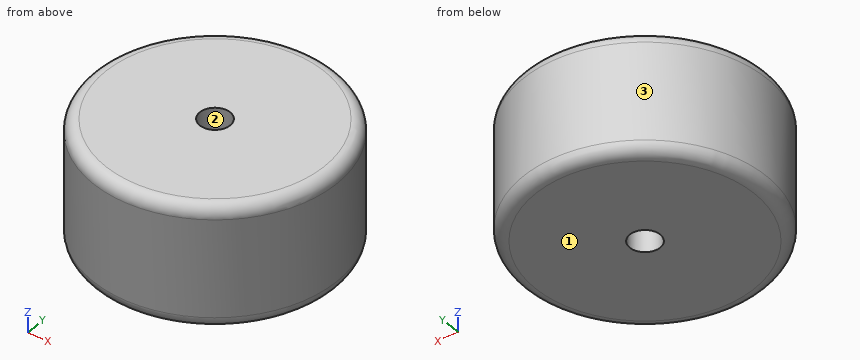
```python
from build123d import *

# Parameters (mm, degrees)
SKETCH1_R           = 25.4
BOSS_EXTRUDE1_DEPTH = 25.4
FILLET1_R           = 2.54
CUT_EXTRUDE1_REACH  = 45.994
SKETCH2_R           = 3.175


with BuildPart() as part:
    # Sketch1 → Boss-Extrude1 (new body)
    with BuildSketch(Plane.XY):
        Circle(SKETCH1_R)
    extrude(amount=BOSS_EXTRUDE1_DEPTH)

    # Fillet1
    fillet1_edges = [part.edges().sort_by_distance(p)[0] for p in [
        (-25.4, 0, 0),
        (-25.4, 0, 25.4),
    ]]
    fillet(fillet1_edges, radius=FILLET1_R)

    # Sketch2 → Cut-Extrude1 (cut, up to next)
    with BuildSketch(Plane.XY.offset(25.4), mode=Mode.PRIVATE) as cut_extrude1_sk1:
        Circle(SKETCH2_R)
    cut_extrude1_tool1 = extrude(cut_extrude1_sk1.sketch, amount=-CUT_EXTRUDE1_REACH, mode=Mode.PRIVATE) & part.part
    add(cut_extrude1_tool1.solids().sort_by_distance((0, 0, 25.4))[0], mode=Mode.SUBTRACT)


solid = part.part
```
Geometry: final body of the model. Coordinates: model frame, mm. Face numbers are marked on the shaded views. Coordinates: 2 decimals unless noted, no trailing zeros. Order: outer loops, then holes, each group sorted by start corner. A loop starts at its lowest first (then second) coordinate and runs counter-clockwise, first axis right, second up. Notation, with made-up numbers: (-23.5, -17.75) - (0.5, -17.75) arc R21 ccw to (0.5, 1.25) - close; hole circle Ø9 at (77, -36). An arc over 180 degrees is marked (long way). Return JSON: item names as keys, results as strings. Group by question number.
1. Cut plane A-A (x = 0). Output: boundary loops of the cut face in (y, z) (3 decimals).
2. Cut plane C-C (z = 10.5). Output: boundary loops of the cut face in (x, y) (3 decimals).
3. Pull-direction query (Y, two-part tool) for the marked faces 1, 2 and 3; classes: pulls with the +Y half, pulls with the -Y half, needs draft (parallel to the pull), parting line crosses it, or undercut.
4. Pin query (flat end, axial travel): pin 1 (4 mm diameter, centred on x = 6, z = 4.5, fed in from -Y); pin 2 (10 mm diameter, centred on y = -15.5, z = 15, fed in from -X); pin 3 (1.5 mm diameter, centred on x = -0.5, z = 14, fed in from +Y). Return the tip coordinate at first contact, or that it passes through.
5. Material intervals for line 1 along Y through (x, z) = (0, 6.75) (3 decimals); line 2 along X through (y, z) = (-2, 21); line 3 along X through (y, z) = (-1.5, 10.75), sorted ascending. Write a range as [from, to].
Resolved:
{
 "1": {"outline": "(-25.4, 2.54) arc R2.54 ccw to (-22.86, 0) - (-3.175, 0) - (-3.175, 25.4) - (-22.86, 25.4) arc R2.54 ccw to (-25.4, 22.86) - close; (3.175, 0) - (22.86, 0) arc R2.54 ccw to (25.4, 2.54) - (25.4, 22.86) arc R2.54 ccw to (22.86, 25.4) - (3.175, 25.4) - close"},
 "2": {"outline": "circle Ø50.8 at (0, 0); hole circle Ø6.35 at (0, 0)"},
 "3": {"face 1": "needs draft", "face 2": "undercut", "face 3": "parting line crosses it"},
 "4": {"pin 1": "stops at y = -25.08", "pin 2": "stops at x = -23.13", "pin 3": "stops at y = 25.4"},
 "5": {"line 1": "y = [-25.4, -3.175], [3.175, 25.4]", "line 2": "x = [-25.32, -2.47], [2.47, 25.32]", "line 3": "x = [-25.36, -2.8], [2.8, 25.36]"}
}
